Autodesk Inventor part; units mm, degrees
ref_plane "YZ Plane" through (0, 0, 0) normal (1, 0, 0) x (0, 1, 0)
ref_plane "XZ Plane" through (0, 0, 0) normal (0, 1, 0) x (-1, 0, 0)
ref_plane "XY Plane" through (0, 0, 0) normal (0, 0, 1) x (1, 0, 0)
sketch "Sketch1" plane through (0, 0, 0) normal (0, 1, 0) x (-1, 0, 0)
  circle A0 centre (0, 0) radius 22.5
  point P0 (0, -22.5)
  dimension "d0" = 45
extrude "Extrusion1" add sketch "Sketch1" along normal blind 105
sketch "Sketch2" plane through (0, 105, 0) normal (0, 1, 0) x (1, 0, 0)
  circle A0 centre (0, -13.247) radius 5
  circle A1 centre (0, 13.247) radius 5
  point P0 (0, 0)
  dimension "d3" = 10
  dimension "d4" = 10
  dimension "d5" = 13.247
  dimension "d6" = 13.247
extrude "Extrusion2" add sketch "Sketch2" along normal blind 10
properties part number "capacitor"
Design review of the part built by this model. Coordinates are the model's own, in mm. A direction names the side the tool comes from. Coordinates: 2 decimals unless noted, no trailing zeros. Loops run counter-clockwise (first coordinate to the right, second up) from the corner with the lowest first, then second, coordinate; pieces in that order, holes last. Notation, with made-up numbers: M -21.75,-21.75 L 31.25,-21.75 A18 ccw 31.25,-12.75 Z; hole C 74.25,47.5 d4. An arc over 180 degrees is marked long. Use one line per item in the form item = value.
(1) Draft analysis for pull direction Z (two halves, no side actions). For faces 1 (the face through (-0.65, 109.93, -8.29)), 2 (the face through (-10.382, 51.765, 19.961)), 3 (the face through (0, 0, 0)), state which applies: pulls with the +Z half, pulls with the -Z half, needs draft (parallel to the pull), parting line crosses it, or undercut.
Return value:
face_1 = undercut
face_2 = parting line crosses it
face_3 = needs draft
(2) For faces 4 (the face through (0, 105, 0)), 5 (the face through (0, 115, 13)), list the 3-axis set-ups (+Z, -Z, +X, -X, +Y, -Y) from which the entire face can be reached by the end or side of a thin tool; tool diameter is ignored.
Return value:
face_4 = +Y
face_5 = +Z, -Z, +X, -X, +Y
(3) Consider section B-B (y = 35). Write out the cut boundary in (x, z), and give its area (3 significant figures).
Return value:
outline = C 0,0 d45
area = 1,590 mm2
(4) Consider section A-A (x = 0). Write out the cut boundary in (y, z).
Return value:
outline = M 0,-22.5 L 105,-22.5 L 105,-18.25 L 115,-18.25 L 115,-8.25 L 105,-8.25 L 105,8.25 L 115,8.25 L 115,18.25 L 105,18.25 L 105,22.5 L 0,22.5 Z
(5) Consider section C-C (z = 0). Write out the cut boundary in (x, y).
Return value:
outline = M -22.5,0 L 22.5,0 L 22.5,105 L -22.5,105 Z
(6) For line 1 along X through (y, z) = (44, -1); line 2 along Y through (x, z) = (13, 9); line 3 along Z through (x, y) = (-0.5, 83.5), list the stretches that pass through material, from the lowest coordinate up. Write a range as from..to.
Return value:
line_1 = -22.48..22.48
line_2 = 0..105
line_3 = -22.49..22.49
(7) Consider section D-D (z = 12). Write out the cut boundary in (x, y), and give its area (3 significant figures).
Return value:
outline = M -19.03,0 L 19.03,0 L 19.03,105 L 4.84,105 L 4.84,115 L -4.84,115 L -4.84,105 L -19.03,105 Z
area = 4,090 mm2
(8) Clearance check with flat-ended pins moving along their axes: P1, Ø4, axis at x = 4, y = 14.5, coming from the +Z side; P2, Ø12, axis at y = 79.5, z = 2, coming from the +X side; P3, Ø1, axis at y = 98, z = 14, coming from the +X side; P4, Ø3, axis at y = 95.5, z = -14.5, coming from the -X side. State where each tip first meets the part, or that it passes through.
Return value:
P1 = 22.41
P2 = 22.5
P3 = 18
P4 = -18.36
